Work out the finished part from the listing and answer in its coordinate system (mm). Give positions to 0.01 mm unless a question says otherwise; leave off trailing zeros. Loops run counter-clockwise (first coordinate to the right, second up) from the corner with the lowest first, then second, coordinate; pieces in that order, holes last. Notation, with made-up numbers: (85.5, -25) - (113.5, -25) arc R5 cw to (113.5, -19) - close; hole circle Ø9 at (80.25, 14.5). An arc over 180 degrees is marked (long way). Use one line per item in the form item = value. Start each with the question number.
from build123d import *

# Parameters (mm, degrees)
F1_DEPTH = 9.525
F3_R     = 5.08


with BuildPart() as f1:
    # F0 (on Front) → F1 (new body)
    with BuildSketch(Plane.XZ):
        with BuildLine():
            Line((0, 101.6), (0, 0))
            Line((0, 0), (19.05, 0))
            Line((19.05, 0), (19.05, 15.6718))
            ThreePointArc((19.05, 15.6718), (15.6718, 19.05), (19.05, 22.4282))
            Line((19.05, 22.4282), (19.05, 53.7718))
            ThreePointArc((19.05, 53.7718), (15.6718, 57.15), (19.05, 60.5282))
            Line((19.05, 60.5282), (19.05, 87.3125))
            ThreePointArc((19.05, 87.3125), (8.947212, 91.497212), (4.7625, 101.6))
            Line((4.7625, 101.6), (0, 101.6))
        make_face()
        with BuildLine():
            Line((19.05, 15.6718), (19.05, 0))
            Line((19.05, 0), (38.1, 0))
            Line((38.1, 0), (38.1, 101.6))
            Line((38.1, 101.6), (33.3375, 101.6))
            ThreePointArc((33.3375, 101.6), (29.152788, 91.497212), (19.05, 87.3125))
            Line((19.05, 87.3125), (19.05, 60.5282))
            ThreePointArc((19.05, 60.5282), (21.438748, 59.538748), (22.4282, 57.15))
            ThreePointArc((22.4282, 57.15), (21.438748, 54.761252), (19.05, 53.7718))
            Line((19.05, 53.7718), (19.05, 22.4282))
            ThreePointArc((19.05, 22.4282), (21.438748, 21.438748), (22.4282, 19.05))
            ThreePointArc((22.4282, 19.05), (21.438748, 16.661252), (19.05, 15.6718))
        make_face()
        with BuildLine():
            ThreePointArc((38.1, 101.6), (19.05, 120.65), (0, 101.6))
            Line((0, 101.6), (4.7625, 101.6))
            ThreePointArc((4.7625, 101.6), (19.05, 115.8875), (33.3375, 101.6))
            Line((33.3375, 101.6), (38.1, 101.6))
        make_face()
    extrude(amount=-F1_DEPTH)

    # F3
    f3_edges = [f1.edges().sort_by_distance(p)[0] for p in [
        (38.1, 4.7625, 0),
        (0, 4.7625, 0),
    ]]
    fillet(f3_edges, radius=F3_R)


solid = f1.part
1) Determine the mould class of faces 1 (the cylindrical face through (1.449, 4.829, 1.528)), 2 (the flat face through (19, 9.525, 48)), 3 (the cylindrical face through (19.469, 4.696, 120.645)), 4 (the flat face through (38.1, 5, 53)) for opening direction X: released by +X, released by -X, zero draft, split by the parting line, or undercut.
2) A cutting plane is placed at B-B (z = 98). Give the vertices of the cut face in (x, y) (3 decimals), plus the area to 3 significant figures.
3) A flat-ended cylindrical pin translates along its axis: pin 1 Ø3 at (x, z) = (8.5, 31) entering from -Y. Find the tip coordinate at first contact, or state that the pin passes through.
4) A cutting plane is placed at C-C (x = 31). Give the vertices of the cut face in (y, z) (3 decimals).
5) Find the intervals of material crossed by probe 1 along Z at (x, y) = (21, 1.75); probe 2 along X at (y, z) = (7.75, 93.5); probe 3 along Z at (x, y) = (11.5, 8.75), in increasing order.
6) A cutting plane is placed at A-A (y = 7.25). State how many separate pieces and enclosed holes the cut face has, plus the area to 3 significant figures.
Answer sheet:
q1.face_1 = released by -X
q1.face_2 = zero draft
q1.face_3 = split by the parting line
q1.face_4 = released by +X
q2.outline = (0, 0) - (5.223, 0) - (5.223, 9.525) - (0, 9.525) - close; (32.877, 0) - (38.1, 0) - (38.1, 9.525) - (32.877, 9.525) - close
q2.area = 99.5 mm²
q3.pin_1 = 0
q4.outline = (0, 0) - (9.525, 0) - (9.525, 93.769) - (0, 93.769) - close; (0, 109.431) - (9.525, 109.431) - (9.525, 116.436) - (0, 116.436) - close
q5.probe_1 = 0 to 16.29, 21.81 to 54.39, 59.91 to 87.45, 115.75 to 120.55
q5.probe_2 = 0 to 7.28, 30.82 to 38.1
q5.probe_3 = 0 to 89.47, 113.73 to 119.09
q6.separate_pieces = 1
q6.enclosed_holes = 3
q6.area = 3,720 mm²
